Here's how the part is built. I have some questions about the finished solid (model axes, mm). A direction names the side the tool comes from. Give positions to 0.01 mm unless a question says otherwise; leave off trailing zeros. Loops run counter-clockwise (first coordinate to the right, second up) from the corner with the lowest first, then second, coordinate; pieces in that order, holes last. Notation, with made-up numbers: (32.25, 14.25) -> (38.25, 14.25) arc R17 cw to (38.25, 20.25) -> close; hole circle Ø9 at (-6.75, 43). An arc over 180 degrees is marked (long way). Answer in a Markdown table with one row per item. Add a question column.
Item 1: If we section it at C-C (z = 27): Write out the boundary of the cut face in (x, y).
Item 2: If we section it at B-B (x = 0): Write out the boundary of the cut face in (y, z), then the cut area to 3 significant figures.
Item 3: For P1, Ø2, axis at x = -0.5, z = 12.5, coming from the -Y side; P2, Ø4, axis at y = -5, z = 28, coming from the -X side; P3, Ø8, axis at y = -5, z = 11.5, coming from the -X side, each with a flat end and sliding along its axis, tell me the tip position at first contact or that it passes through.
Item 4: Which directions (+Z, -Z, +X, -X, +Y, -Y) give clear straight access to the entire face, cutting with the end or side of a thin tool? Please do faces 1 (the face through (4, -6, 39)), 2 (the face through (-10.493, 0.382, 1.972)).
Item 5: If we section it at A-A (y = 0): Write out the boundary of the cut face in (x, z), then the cut area to 3 significant figures.
Item 6: If I drill on line 1 (Z direction, x = 3.5, y = 9.75); line 2 (Y direction, x = 0.25, z = 11), over which ranges is the centre line in solid material (lowest first)?
Item 7: If we section it at D-D (z = 40.5): Write out the boundary of the cut face in (x, y).
```python
from build123d import *

# Parameters (mm, degrees)
F0_R     = 10.5
F1_DEPTH = 4
F2_R     = 8
F3_DEPTH = 39
F4_W     = 7
F4_H     = 5
F6_W     = 5.926284
F6_H     = 21.135783
F7_DEPTH = 6


with BuildPart() as f1:
    # F0 (on Top) → F1 (new body)
    with BuildSketch(Plane.XY):
        Circle(F0_R)
    extrude(amount=F1_DEPTH)

    # F2 (on Top) → F3 (join)
    with BuildSketch(Plane.XY):
        Circle(F2_R)
    extrude(amount=F3_DEPTH)

    # F4 (on Right) → F5 (revolve)
    with BuildSketch(Plane.YZ):
        with Locations((3.5, 41.5)):
            Rectangle(F4_W, F4_H)
    revolve(axis=Axis((0, 0, 41.5), (0, 0, -1)))

    # F6 (on Top) → F7 (cut)
    with BuildSketch(Plane.XY):
        with Locations((11.963142, 0.046621)):
            Rectangle(F6_W, F6_H)
    extrude(amount=F7_DEPTH, mode=Mode.SUBTRACT)


solid = f1.part
```
Recorded:
| question | item | result |
|---|---|---|
| 1 | outline | circle Ø16 at (0, 0) |
| 2 | outline | (-10.5, 0) -> (10.5, 0) -> (10.5, 4) -> (8, 4) -> (8, 39) -> (7, 39) -> (7, 44) -> (-7, 44) -> (-7, 39) -> (-8, 39) -> (-8, 4) -> (-10.5, 4) -> close |
| 2 | area | 714 mm^2 |
| 3 | P1 | stops at y = -8 |
| 3 | P2 | stops at x = -7.42 |
| 3 | P3 | stops at x = -7.94 |
| 4 | face 1 | +Z |
| 4 | face 2 | +Z, -Z |
| 5 | outline | (-10.5, 0) -> (9, 0) -> (9, 4) -> (8, 4) -> (8, 39) -> (7, 39) -> (7, 44) -> (-7, 44) -> (-7, 39) -> (-8, 39) -> (-8, 4) -> (-10.5, 4) -> close |
| 5 | area | 708 mm^2 |
| 6 | line 1 | z = 0 to 4 |
| 6 | line 2 | y = -8 to 8 |
| 7 | outline | circle Ø14 at (0, 0) |
